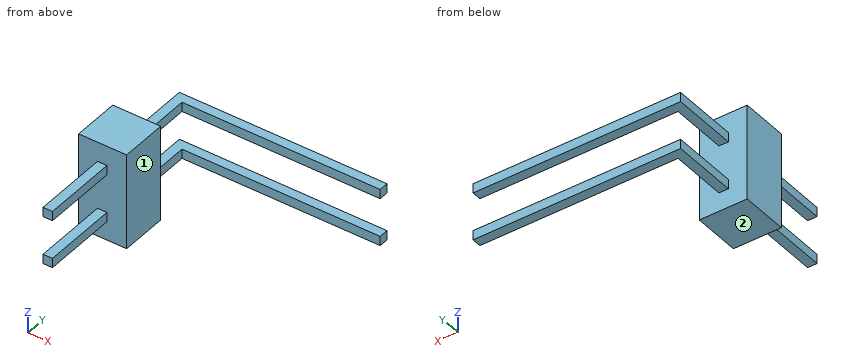
from build123d import *

# Parameters (mm, degrees)
BOSS_EXTRU_1_DEPTH         = 0.5
ESQUISSE2_W                = 2.54
ESQUISSE2_H                = 2.54
BOSS_EXTRU_2_DEPTH         = 2.5
R_P_TITION_LIN_AIRE3_COUNT = 2
R_P_TITION_LIN_AIRE3_PITCH = 2.54


with BuildPart() as part:
    # Esquisse1 → Boss.-Extru.1 (new body)
    with BuildSketch(Plane.XY):
        Polygon((0, -4), (0, 6), (11, 6), (11, 5.5), (0.5, 5.5), (0.5, -4), align=None)
    boss_extru_1 = extrude(amount=BOSS_EXTRU_1_DEPTH)

    # Esquisse2 → Boss.-Extru.2 (add)
    with BuildSketch(Plane(origin=(0, 0, 0), x_dir=(1, 0, 0), z_dir=(0, 1, 0))):
        with Locations((0.27, -0.27)):
            Rectangle(ESQUISSE2_W, ESQUISSE2_H)
    boss_extru_2 = extrude(amount=BOSS_EXTRU_2_DEPTH)

    # Répétition linéaire3: Boss.-Extru.1, Boss.-Extru.2 ×2
    with Locations(*[(0, 0, i * R_P_TITION_LIN_AIRE3_PITCH) for i in range(1, R_P_TITION_LIN_AIRE3_COUNT)]):
        add(boss_extru_1)
        add(boss_extru_2)


solid = part.part
Input: part model. Units: mm. Frame: model coordinates. Face numbers are marked on the shaded views. A direction names the side the tool comes from. Coordinates: 2 decimals unless noted, no trailing zeros. Order: outer loops, then holes, each group sorted by start corner. A loop starts at its lowest first (then second) coordinate and runs counter-clockwise, first axis right, second up. Notation, with made-up numbers: M -2.75,53.5 L 15.25,53.5 A22 cw 15.25,59.5 Z; hole C -28,32 d11. An arc over 180 degrees is marked long. Answer in a Markdown table with one row per item.
(1) Section query B-B, the plane y = 3.5. Output: boundary loops of the cut face in (x, z).
Numbers:
| item | result |
|---|---|
| outline | M 0,0 L 0.5,0 L 0.5,0.5 L 0,0.5 Z; M 0,2.54 L 0.5,2.54 L 0.5,3.04 L 0,3.04 Z |
(2) Contact query for flat-ended pins moving along their axis: pin 1 Ø0.8 at (x, z) = (0, 1) entering from +Y; pin 2 Ø3 at (y, z) = (1.5, 1) entering from +X; pin 3 Ø3 at (x, y) = (5, 5) entering from +Z; pin 4 Ø1 at (x, y) = (7, 3.5) entering from -Z. Output: stop coordinate, or through.
Numbers:
| item | result |
|---|---|
| pin 1 | stops at y = 2.5 |
| pin 2 | stops at x = 1.54 |
| pin 3 | stops at z = 3.04 |
| pin 4 | passes through |
(3) Section query A-A, the plane x = 1.25. Output: boundary loops of the cut face in (y, z).
Numbers:
| item | result |
|---|---|
| outline | M 0,-1 L 2.5,-1 L 2.5,4.08 L 0,4.08 Z; M 5.5,0 L 6,0 L 6,0.5 L 5.5,0.5 Z; M 5.5,2.54 L 6,2.54 L 6,3.04 L 5.5,3.04 Z |
(4) Section query C-C, the plane x = 9.25. Output: boundary loops of the cut face in (y, z).
Numbers:
| item | result |
|---|---|
| outline | M 5.5,0 L 6,0 L 6,0.5 L 5.5,0.5 Z; M 5.5,2.54 L 6,2.54 L 6,3.04 L 5.5,3.04 Z |
(5) Material intervals for line 1 (Z direction, x = 7.75, y = 5.75); line 2 (X direction, y = 2, z = 1.1); line 3 (Y direction, x = 0.75, z = 2.65), sorted ascending. Write a range as [from, to].
Numbers:
| item | result |
|---|---|
| line 1 | z = [0, 0.5], [2.54, 3.04] |
| line 2 | x = [-1, 1.54] |
| line 3 | y = [0, 2.5], [5.5, 6] |
(6) Section query D-D, the plane z = 0.3. Output: boundary loops of the cut face in (x, y).
Numbers:
| item | result |
|---|---|
| outline | M -1,0 L 0,0 L 0,-4 L 0.5,-4 L 0.5,0 L 1.54,0 L 1.54,2.5 L 0.5,2.5 L 0.5,5.5 L 11,5.5 L 11,6 L 0,6 L 0,2.5 L -1,2.5 Z |
(7) Access query for the marked faces 1 and 2. Directions: +Z, -Z, +X, -X, +Y, -Y. A direction counts if a zero-diameter tool reaches every point of the face in a straight line with its end or side. Return the directions, or none.
Numbers:
| item | result |
|---|---|
| face 1 | +Z, -Z, +X, -Y |
| face 2 | -Z, +X, -X, +Y, -Y |
